from build123d import *

# Parameters (mm, degrees)
F0_R     = 8.1245
F1_DEPTH = 10
F2_R     = 5


with BuildPart() as f1:
    # F0 (on Top) → F1 (new body)
    with BuildSketch(Plane.XY):
        with BuildLine():
            ThreePointArc((5.016295, 65.530641), (-13.232302, 74.074747), (-8.108205, 54.587401))
            ThreePointArc((-8.108205, 54.587401), (-6.108205, 54.406141), (-4.108205, 54.587401))
            ThreePointArc((-4.108205, 54.587401), (2.435901, 58.406544), (5.016295, 65.530641))
        make_face()
        with Locations((-6.108205, 65.530641)):
            Circle(F0_R, mode=Mode.SUBTRACT)
        with BuildLine():
            Line((-8.108205, 40.99443), (-36.108205, 40.99443))
            ThreePointArc((-36.108205, 40.99443), (-39.643739, 39.529964), (-41.108205, 35.99443))
            Line((-41.108205, 35.99443), (-41.108205, -16.00557))
            ThreePointArc((-41.108205, -16.00557), (-39.643739, -19.541104), (-36.108205, -21.00557))
            Line((-36.108205, -21.00557), (23.891795, -21.00557))
            ThreePointArc((23.891795, -21.00557), (27.427329, -19.541104), (28.891795, -16.00557))
            Line((28.891795, -16.00557), (28.891795, 35.99443))
            ThreePointArc((28.891795, 35.99443), (27.427329, 39.529964), (23.891795, 40.99443))
            Line((23.891795, 40.99443), (-4.108205, 40.99443))
            Line((-4.108205, 40.99443), (-4.108205, 54.587401))
            ThreePointArc((-4.108205, 54.587401), (-6.108205, 54.406141), (-8.108205, 54.587401))
            Line((-8.108205, 54.587401), (-8.108205, 40.99443))
        make_face()
        with BuildLine():
            ThreePointArc((-37.108205, 31.99443), (-35.643739, 35.529964), (-32.108205, 36.99443))
            Line((-32.108205, 36.99443), (19.891795, 36.99443))
            ThreePointArc((19.891795, 36.99443), (23.427329, 35.529964), (24.891795, 31.99443))
            Line((24.891795, 31.99443), (24.891795, -12.00557))
            ThreePointArc((24.891795, -12.00557), (23.427329, -15.541104), (19.891795, -17.00557))
            Line((19.891795, -17.00557), (-32.108205, -17.00557))
            ThreePointArc((-32.108205, -17.00557), (-35.643739, -15.541104), (-37.108205, -12.00557))
            Line((-37.108205, -12.00557), (-37.108205, 31.99443))
        make_face(mode=Mode.SUBTRACT)
    extrude(amount=F1_DEPTH)

    # F2
    f2_edges = [f1.edges().sort_by_distance(p)[0] for p in [
        (-4.108205, 54.587401, 5),
        (-8.108205, 54.587401, 5),
        (-8.108205, 40.99443, 5),
        (-4.108205, 40.99443, 5),
    ]]
    fillet(f2_edges, radius=F2_R)


solid = f1.part
Verification items for the finished model (mm, model axes). A direction names the side the tool comes from. Give positions to 0.01 mm unless a question says otherwise; leave off trailing zeros. Loops run counter-clockwise (first coordinate to the right, second up) from the corner with the lowest first, then second, coordinate; pieces in that order, holes last. Notation, with made-up numbers: (79, 66) - (137, 66) arc R11 cw to (137, 74) - close; hole circle Ø8 at (84, -20.75). An arc over 180 degrees is marked (long way). Write item = value, one per line. Start each with the question number.
Q1. Thickness scan on line 1 (X direction, y = 10.5, z = 4); line 2 (Y direction, x = -28.5, z = 6.75); line 3 (Y direction, x = -6, z = 2.5). Record the ranges inside material, lowest first.
Q2. Cross-section at D-D, the plane x = -3. Enter the section's corners in (y, z), and give its area (3 significant figures).
Q3. Depth check by flat-ended pin: P1, Ø5.5, axis at y = 49.5, z = 4.5, coming from the -X side; P2, Ø2.5, axis at y = 49, z = 5.5, coming from the +X side; P3, Ø5, axis at x = -16, z = 8, coming from the +Y side. Enter the tip coordinate at first touch or a pass-through.
Q4. Cross-section at B-B, the plane y = 13.5. Enter the section's corners in (x, z).
Q5. Tool access check on faces 4 (the face through (-8.895, 53.698, 5.07)), 5 (the face through (-7, -21.006, 5)), 6 (the face through (-6, 36.994, 5)). Record the directions out of +Z, -Z, +X, -X, +Y, -Y that give a thin tool (end or side, any length) a straight path to the whole face; none if there is none.
Q6. Cross-section at C-C, the plane z = 1.25. Enter the section's corners in (x, y), and give its area (3 significant figures).
Q7. Mould release check, pull along X, two halves, no side actions. Record for faces 1 (the face through (-4.108, 48, 5)), 2 (the face through (-9, 39, 0)), 3 (the face through (-6, -17.006, 5)): released by +X, released by -X, zero draft, split by the parting line, or undercut.
Q8. Cross-section at A-A, the plane x = 8.5. Enter the section's corners in (y, z).
Answer key:
q1.line_1 = -41.11 to -37.11, 24.89 to 28.89
q1.line_2 = -21.01 to -17.01, 36.99 to 40.99
q1.line_3 = -21.01 to -17.01, 36.99 to 57.41, 73.65 to 76.65
q2.outline = (-21.01, 0) - (-17.01, 0) - (-17.01, 10) - (-21.01, 10) - close; (36.99, 0) - (42.86, 0) - (42.86, 10) - (36.99, 10) - close; (54.14, 0) - (58.02, 0) - (58.02, 10) - (54.14, 10) - close; (73.04, 0) - (76.21, 0) - (76.21, 10) - (73.04, 10) - close
q2.area = 169 mm^2
q3.P1 = -8.27
q3.P2 = -4.11
q3.P3 = 73.84
q4.outline = (-41.11, 0) - (-37.11, 0) - (-37.11, 10) - (-41.11, 10) - close; (24.89, 0) - (28.89, 0) - (28.89, 10) - (24.89, 10) - close
q5.face_4 = +Z, -Z, -X
q5.face_5 = +Z, -Z, +X, -X, -Y
q5.face_6 = +Z, -Z
q6.outline = (-41.11, -16.01) arc R5 ccw to (-36.11, -21.01) - (23.89, -21.01) arc R5 ccw to (28.89, -16.01) - (28.89, 35.99) arc R5 ccw to (23.89, 40.99) - (0.89, 40.99) arc R5 cw to (-4.11, 45.99) - (-4.11, 51) arc R5 cw to (-1.28, 55.51) arc R11.12 ccw (long way) to (-10.94, 55.51) arc R5 cw to (-8.11, 51) - (-8.11, 45.99) arc R5 cw to (-13.11, 40.99) - (-36.11, 40.99) arc R5 ccw to (-41.11, 35.99) - close; hole (-37.11, -12.01) arc R5 ccw to (-32.11, -17.01) - (19.89, -17.01) arc R5 ccw to (24.89, -12.01) - (24.89, 31.99) arc R5 ccw to (19.89, 36.99) - (-32.11, 36.99) arc R5 ccw to (-37.11, 31.99) - close; hole circle Ø16.25 at (-6.11, 65.53)
q6.area = 1,240 mm^2
q7.face_1 = released by +X
q7.face_2 = zero draft
q7.face_3 = undercut
q8.outline = (-21.01, 0) - (-17.01, 0) - (-17.01, 10) - (-21.01, 10) - close; (36.99, 0) - (40.99, 0) - (40.99, 10) - (36.99, 10) - close
